```python
from build123d import *

# Parameters (mm, degrees)
SKETCH2_R           = 1.65
SKETCH2_R_2         = 1.35
BOSS_EXTRUDE1_DEPTH = 3
SKETCH3_R           = 3
SKETCH3_R_2         = 1.35
BOSS_EXTRUDE2_DEPTH = 2


with BuildPart() as part:
    # Sketch2 → Boss-Extrude1 (new body)
    with BuildSketch(Plane(origin=(0, 0, 0), x_dir=(1, 0, 0), z_dir=(0, 1, 0))):
        with BuildLine():
            Line((-66, 50.5), (52, 50.5))
            ThreePointArc((52, 50.5), (55.535533906, 49.035533906), (57, 45.5))
            Line((57, 45.5), (57, -45.5))
            ThreePointArc((57, -45.5), (55.535533906, -49.035533906), (52, -50.5))
            Line((52, -50.5), (-66, -50.5))
            ThreePointArc((-66, -50.5), (-69.535533906, -49.035533906), (-71, -45.5))
            Line((-71, -45.5), (-71, 45.5))
            ThreePointArc((-71, 45.5), (-69.535533906, 49.035533906), (-66, 50.5))
        make_face()
        with Locations(Location((52, 45.5, 0), (0, 0, 270))):
            Circle(SKETCH2_R, mode=Mode.SUBTRACT)
        with Locations(Location((52, -45.5, 0), (0, 0, 270))):
            Circle(SKETCH2_R, mode=Mode.SUBTRACT)
        with Locations(Location((-66, -45.5, 0), (0, 0, 270))):
            Circle(SKETCH2_R, mode=Mode.SUBTRACT)
        with Locations(Location((-66, 45.5, 0), (0, 0, 270))):
            Circle(SKETCH2_R, mode=Mode.SUBTRACT)
        with Locations(Location((-56, -3.5, 0), (0, 0, 270))):
            Circle(SKETCH2_R_2, mode=Mode.SUBTRACT)
        with Locations(Location((-56, 45.5, 0), (0, 0, 270))):
            Circle(SKETCH2_R_2, mode=Mode.SUBTRACT)
        with Locations(Location((2, 45.5, 0), (0, 0, 270))):
            Circle(SKETCH2_R_2, mode=Mode.SUBTRACT)
        with Locations(Location((2, -3.5, 0), (0, 0, 270))):
            Circle(SKETCH2_R_2, mode=Mode.SUBTRACT)
        with BuildLine():
            Line((12, 40.5), (42, 40.5))
            ThreePointArc((42, 40.5), (45.535533906, 39.035533906), (47, 35.5))
            Line((47, 35.5), (47, 6.5))
            ThreePointArc((47, 6.5), (45.535533906, 2.964466094), (42, 1.5))
            Line((42, 1.5), (12, 1.5))
            ThreePointArc((12, 1.5), (8.464466094, 2.964466094), (7, 6.5))
            Line((7, 6.5), (7, 35.5))
            ThreePointArc((7, 35.5), (8.464466094, 39.035533906), (12, 40.5))
        make_face(mode=Mode.SUBTRACT)
        with BuildLine():
            Line((12, -8.5), (42, -8.5))
            ThreePointArc((42, -8.5), (45.535533906, -9.964466094), (47, -13.5))
            Line((47, -13.5), (47, -35.5))
            ThreePointArc((47, -35.5), (45.535533906, -39.035533906), (42, -40.5))
            Line((42, -40.5), (12, -40.5))
            ThreePointArc((12, -40.5), (8.464466094, -39.035533906), (7, -35.5))
            Line((7, -35.5), (7, -13.5))
            ThreePointArc((7, -13.5), (8.464466094, -9.964466094), (12, -8.5))
        make_face(mode=Mode.SUBTRACT)
        with BuildLine():
            Line((-8, -8.5), (-56, -8.5))
            ThreePointArc((-56, -8.5), (-59.535533906, -9.964466094), (-61, -13.5))
            Line((-61, -13.5), (-61, -35.5))
            ThreePointArc((-61, -35.5), (-59.535533906, -39.035533906), (-56, -40.5))
            Line((-56, -40.5), (-8, -40.5))
            ThreePointArc((-8, -40.5), (-4.464466094, -39.035533906), (-3, -35.5))
            Line((-3, -35.5), (-3, -13.5))
            ThreePointArc((-3, -13.5), (-4.464466094, -9.964466094), (-8, -8.5))
        make_face(mode=Mode.SUBTRACT)
        with BuildLine():
            Line((-46, 43), (-8, 43))
            ThreePointArc((-8, 43), (-4.464466094, 41.535533906), (-3, 38))
            Line((-3, 38), (-3, 6.5))
            ThreePointArc((-3, 6.5), (-4.464466094, 2.964466094), (-8, 1.5))
            Line((-8, 1.5), (-46, 1.5))
            ThreePointArc((-46, 1.5), (-49.535533906, 2.964466094), (-51, 6.5))
            Line((-51, 6.5), (-51, 38))
            ThreePointArc((-51, 38), (-49.535533906, 41.535533906), (-46, 43))
        make_face(mode=Mode.SUBTRACT)
    extrude(amount=BOSS_EXTRUDE1_DEPTH)

    # Sketch3 → Boss-Extrude2 (add)
    # profile 1 of 4: a face of its own
    with BuildSketch(Plane(origin=(0, 3, 0), x_dir=(1, 0, 0), z_dir=(0, 1, 0))):
        with Locations(Location((-56, -3.5, 0), (0, 0, 270))):
            Circle(SKETCH3_R)
        with Locations(Location((-56, -3.5, 0), (0, 0, 270))):
            Circle(SKETCH3_R_2, mode=Mode.SUBTRACT)
    # profile 2 of 4: a face of its own
    with BuildSketch(Plane(origin=(0, 3, 0), x_dir=(1, 0, 0), z_dir=(0, 1, 0))):
        with Locations(Location((2, -3.5, 0), (0, 0, 270))):
            Circle(SKETCH3_R)
        with Locations(Location((2, -3.5, 0), (0, 0, 270))):
            Circle(SKETCH3_R_2, mode=Mode.SUBTRACT)
    # profile 3 of 4: a face of its own
    with BuildSketch(Plane(origin=(0, 3, 0), x_dir=(1, 0, 0), z_dir=(0, 1, 0))):
        with Locations(Location((2, 45.5, 0), (0, 0, 270))):
            Circle(SKETCH3_R)
        with Locations(Location((2, 45.5, 0), (0, 0, 270))):
            Circle(SKETCH3_R_2, mode=Mode.SUBTRACT)
    # profile 4 of 4: a face of its own
    with BuildSketch(Plane(origin=(0, 3, 0), x_dir=(1, 0, 0), z_dir=(0, 1, 0))):
        with Locations(Location((-56, 45.5, 0), (0, 0, 270))):
            Circle(SKETCH3_R)
        with Locations(Location((-56, 45.5, 0), (0, 0, 270))):
            Circle(SKETCH3_R_2, mode=Mode.SUBTRACT)
    extrude(amount=BOSS_EXTRUDE2_DEPTH)


solid = part.part
```
Source: CAD feature listing. Evaluate the final solid. Frame: model axes, mm. A direction names the side the tool comes from. Round coordinates to 2 decimals unless told otherwise and drop trailing zeros. Loops run counter-clockwise (first coordinate to the right, second up) from the corner with the lowest first, then second, coordinate; pieces in that order, holes last. Notation, with made-up numbers: M 5.25,76 L 12.25,76 A27 ccw 12.25,105 Z; hole C 52,24 d2. An arc over 180 degrees is marked long. Use a Markdown table: item, result. Add a question column.
1. Set-up query: faces 1 (the cylindrical face through (-53.026, 3.986, -45.891)), 2 (the cylindrical face through (-49.5, 1.48, -2.93)), 3 (the cylindrical face through (-69.5, 1.48, 49.07)). Return all of +Z, -Z, +X, -X, +Y, -Y with unobstructed straight access to the full face (end or side cutting, diameter ignored); none if empty.
2. Cut plane A-A, the plane z = 3.5. Output: boundary loops of the cut face in (x, y), and give its area (3 significant figures).
3. Cut plane D-D, the plane x = 19. Output: boundary loops of the cut face in (y, z), and give its area (3 significant figures).
4. Cut plane B-B, the plane x = 2. Output: boundary loops of the cut face in (y, z), and give its area (3 significant figures).
5. Contact query for a flat-ended pin moving along its axis: pin 1 (4 mm diameter, centred on x = 52, z = -45.5, fed in from +Y). Output: stop coordinate, or through.
6. Ray query, line 1 along Z through (x, y) = (12.5, 0.8); line 2 along X through (y, z) = (2.65, -36); line 3 along X through (y, z) = (1.25, 45.5). Return the intervals inside material, ascending. Write a range as [from, to].
7. Cut plane C-C, the plane z = -26. Output: boundary loops of the cut face in (x, y).
8. Pull-direction query (Z, two-part tool) for faces 4 (the cylindrical face through (-69.57, 1.48, -49)), 5 (the flat face through (-57, 5, -44)), 6 (the cylindrical face through (-53.026, 3.986, 3.109)); classes: +Z half, -Z half, draft (parallel to the pull), parting line (faces both ways), or undercut.
Solution:
| question | item | result |
|---|---|---|
| 1 | face 1 | +Y |
| 1 | face 2 | +Y, -Y |
| 1 | face 3 | +Z, -X, +Y, -Y |
| 2 | outline | M -71,0 L -57.35,0 L -57.35,5 L -59,5 L -59,3 L -71,3 Z; M -54.65,0 L 0.65,0 L 0.65,5 L -1,5 L -1,3 L -53,3 L -53,5 L -54.65,5 Z; M 3.35,0 L 57,0 L 57,3 L 5,3 L 5,5 L 3.35,5 Z |
| 2 | area | 381 mm2 |
| 3 | outline | M 0,-50.5 L 3,-50.5 L 3,-40.5 L 0,-40.5 Z; M 0,-1.5 L 3,-1.5 L 3,8.5 L 0,8.5 Z; M 0,40.5 L 3,40.5 L 3,50.5 L 0,50.5 Z |
| 3 | area | 90.0 mm2 |
| 4 | outline | M 0,-50.5 L 3,-50.5 L 3,-48.5 L 5,-48.5 L 5,-46.85 L 0,-46.85 Z; M 0,-44.15 L 5,-44.15 L 5,-42.5 L 3,-42.5 L 3,0.5 L 5,0.5 L 5,2.15 L 0,2.15 Z; M 0,4.85 L 5,4.85 L 5,6.5 L 3,6.5 L 3,50.5 L 0,50.5 Z |
| 4 | area | 300 mm2 |
| 5 | pin 1 | stops at y = 3 |
| 6 | line 1 | z = [-50.5, -40.5], [-1.5, 8.5], [40.5, 50.5] |
| 6 | line 2 | x = [-71, -51], [-3, 7.03], [46.97, 57] |
| 6 | line 3 | x = [-71, -67.65], [-64.35, 50.35], [53.65, 57] |
| 7 | outline | M -71,0 L -51,0 L -51,3 L -71,3 Z; M -3,0 L 7,0 L 7,3 L -3,3 Z; M 47,0 L 57,0 L 57,3 L 47,3 Z |
| 8 | face 4 | -Z half |
| 8 | face 5 | draft |
| 8 | face 6 | undercut |
